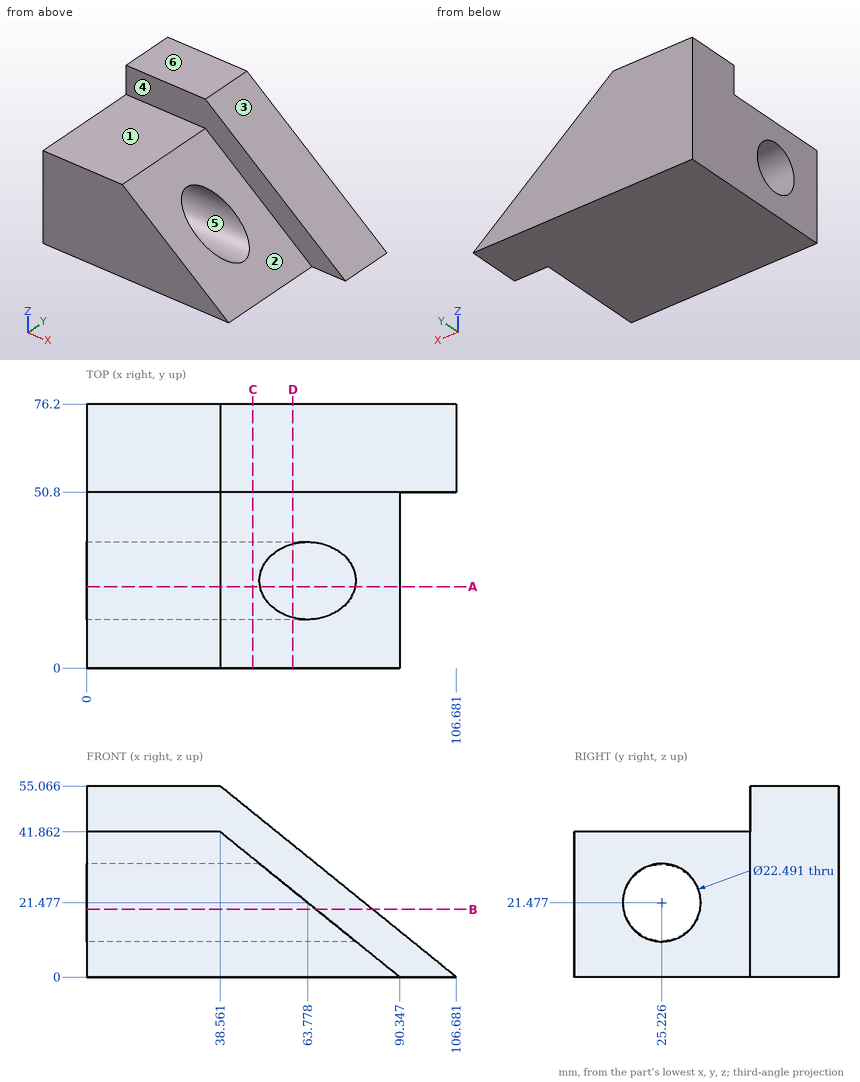
Job drawing, mm, ordinate dimensions from the low corner. One solid piece. A direction names the side the tool comes from. Round coordinates to 2 decimals unless told otherwise and drop trailing zeros. Loops run counter-clockwise (first coordinate to the right, second up) from the corner with the lowest first, then second, coordinate; pieces in that order, holes last.
(1) Wall check: line 1 along Y through (x, z) = (72.5, 17.5); line 2 along Z through (x, y) = (36, 4); line 3 along X through (y, z) = (41.5, 25). Give the ranges that are in metal, low to high.
(2) Cut at D-D (x = 59.5). Give the cut face in (y, z) (1 decimal).
(3) Cut at C-C (x = 48). Give the cut face in (y, z) (1 decimal).
(4) Cut at B-B (z = 19.5). Give the cut face in (x, y) (1 decimal), plus the area to 4 significant figures.
(5) Which spindle directions (+Z, -Z, +X, -X, +Y, -Y) get a long thin tool onto all of the face, cutting with end or side? Do the marked faces 1, 2 and 3. Say none if no direction does.
(6) Cut at A-A (y = 23.5). Give the cut face in (x, z) (1 decimal).
(7) Two-plate mould, pull along Y, no slides. Class the marked faces 4, 5 and 6: +Y half, -Y half, draft (parallel to the pull), parting line (faces both ways), or undercut.
(8) Drop flat-ended pins along their axis: pin 1 (10 mm diameter, centred on y = 29.5, z = 6.5, fed in from +X); pin 2 (6 mm diameter, centred on x = 87, y = 43, fed in from +Z); pin 3 (13.5 mm diameter, centred on y = 25.23, z = 21.48, fed in from +X); pin 4 (8 mm diameter, centred on x = 21.5, y = 26.5, fed in from +Z). Give the stop position or say it passes through.
Findings below:
1. line 1: y = 50.8 to 76.2
1. line 2: z = 0 to 41.86
1. line 3: x = 0 to 59.42
2. outline: (0, 0) - (76.2, 0) - (76.2, 38.1) - (50.8, 38.1) - (50.8, 24.9) - (35.9, 24.9) arc R11.2 cw (long way) to (14.5, 24.9) - (0, 24.9) - close
3. outline: (0, 0) - (76.2, 0) - (76.2, 47.4) - (50.8, 47.4) - (50.8, 34.2) - (0, 34.2) - close; hole circle Ø22.5 at (25.2, 21.5)
4. outline: (0, 0) - (66.2, 0) - (66.2, 14.2) - (0, 14.2) - close; (0, 36.3) - (66.2, 36.3) - (66.2, 50.8) - (82.6, 50.8) - (82.6, 76.2) - (0, 76.2) - close
4. area: 3,995 mm2
5. face 1: +Z, +X, -X, -Y
5. face 2: +Z, +X, -Y
5. face 3: +Z, +X, +Y, -Y
6. outline: (0, 0) - (90.3, 0) - (77.5, 10.4) - (0, 10.4) - close; (0, 32.6) - (50, 32.6) - (38.6, 41.9) - (0, 41.9) - close
7. face 4: -Y half
7. face 5: undercut
7. face 6: draft
8. pin 1: stops at x = 88.49
8. pin 2: stops at z = 5.13
8. pin 3: passes through
8. pin 4: stops at z = 41.86
